from build123d import *

# Parameters (mm, degrees)
BOSS_EXTRUDE1_DEPTH = 23
CUT_EXTRUDE1_REACH  = 53.631
SKETCH4_R           = 1.95
CUT_EXTRUDE3_REACH  = 59.631
CUT_EXTRUDE3_START  = -6
CUT_EXTRUDE4_REACH  = 65.269
SKETCH7_R           = 2.75
CUT_EXTRUDE5_REACH  = 85.269
CUT_EXTRUDE5_START  = -20
SKETCH8_R           = 5
FILLET1_R           = 4


with BuildPart() as part:
    # Sketch3 → Boss-Extrude1 (new, symmetric)
    with BuildSketch(Plane(origin=(0, 0, 0), x_dir=(0, 0, -1), z_dir=(1, 0, 0))):
        Polygon((31.368752944, 7.9863551), (20.770501764, 0), (30, 0), (30, -6), (-30, -6), (-30, 0), (-20.770501764, 0), (16.323377365, 27.952242852), align=None)
    extrude(amount=BOSS_EXTRUDE1_DEPTH, both=True)

    # Sketch4 → Cut-Extrude1 (cut, up to next)
    with BuildSketch(Plane(origin=(0, -6, 0), x_dir=(-1, 0, 0), z_dir=(0, -1, 0)), mode=Mode.PRIVATE) as cut_extrude1_sk1:
        with Locations(Location((15, 15, 0), (0, 0, 90))):
            Circle(SKETCH4_R)
    cut_extrude1_tool1 = extrude(cut_extrude1_sk1.sketch, amount=-CUT_EXTRUDE1_REACH, mode=Mode.PRIVATE) & part.part
    # Sketch4 → Cut-Extrude1 (cut, up to next)
    with BuildSketch(Plane(origin=(0, -6, 0), x_dir=(-1, 0, 0), z_dir=(0, -1, 0)), mode=Mode.PRIVATE) as cut_extrude1_sk2:
        with Locations(Location((15, -15, 0), (0, 0, 90))):
            Circle(SKETCH4_R)
    cut_extrude1_tool2 = extrude(cut_extrude1_sk2.sketch, amount=-CUT_EXTRUDE1_REACH, mode=Mode.PRIVATE) & part.part
    # Sketch4 → Cut-Extrude1 (cut, up to next)
    with BuildSketch(Plane(origin=(0, -6, 0), x_dir=(-1, 0, 0), z_dir=(0, -1, 0)), mode=Mode.PRIVATE) as cut_extrude1_sk3:
        with Locations(Location((-15, -15, 0), (0, 0, 90))):
            Circle(SKETCH4_R)
    cut_extrude1_tool3 = extrude(cut_extrude1_sk3.sketch, amount=-CUT_EXTRUDE1_REACH, mode=Mode.PRIVATE) & part.part
    # Sketch4 → Cut-Extrude1 (cut, up to next)
    with BuildSketch(Plane(origin=(0, -6, 0), x_dir=(-1, 0, 0), z_dir=(0, -1, 0)), mode=Mode.PRIVATE) as cut_extrude1_sk4:
        with Locations(Location((-15, 15, 0), (0, 0, 90))):
            Circle(SKETCH4_R)
    cut_extrude1_tool4 = extrude(cut_extrude1_sk4.sketch, amount=-CUT_EXTRUDE1_REACH, mode=Mode.PRIVATE) & part.part
    add(cut_extrude1_tool1.solids().sort_by_distance((-15, -6, -15))[0], mode=Mode.SUBTRACT)
    add(cut_extrude1_tool2.solids().sort_by_distance((-15, -6, 15))[0], mode=Mode.SUBTRACT)
    add(cut_extrude1_tool3.solids().sort_by_distance((15, -6, 15))[0], mode=Mode.SUBTRACT)
    add(cut_extrude1_tool4.solids().sort_by_distance((15, -6, -15))[0], mode=Mode.SUBTRACT)

    # Sketch6 → Cut-Extrude3 (cut, up to next)
    with BuildSketch(Plane(origin=(0, -6, 0), x_dir=(-1, 0, 0), z_dir=(0, -1, 0)).offset(CUT_EXTRUDE3_START), mode=Mode.PRIVATE) as cut_extrude3_sk1:
        Polygon((-15, -18.983716857), (-18.45, -16.991858429), (-18.45, -13.008141571), (-15, -11.016283143), (-11.55, -13.008141571), (-11.55, -16.991858429), align=None)
    cut_extrude3_tool1 = extrude(cut_extrude3_sk1.sketch, amount=-CUT_EXTRUDE3_REACH, mode=Mode.PRIVATE) & part.part
    # Sketch6 → Cut-Extrude3 (cut, up to next)
    with BuildSketch(Plane(origin=(0, -6, 0), x_dir=(-1, 0, 0), z_dir=(0, -1, 0)).offset(CUT_EXTRUDE3_START), mode=Mode.PRIVATE) as cut_extrude3_sk2:
        Polygon((18.45, -16.991858429), (18.45, -13.008141571), (15, -11.016283143), (11.55, -13.008141571), (11.55, -16.991858429), (15, -18.983716857), align=None)
    cut_extrude3_tool2 = extrude(cut_extrude3_sk2.sketch, amount=-CUT_EXTRUDE3_REACH, mode=Mode.PRIVATE) & part.part
    # Sketch6 → Cut-Extrude3 (cut, up to next)
    with BuildSketch(Plane(origin=(0, -6, 0), x_dir=(-1, 0, 0), z_dir=(0, -1, 0)).offset(CUT_EXTRUDE3_START), mode=Mode.PRIVATE) as cut_extrude3_sk3:
        Polygon((15, 11.016283143), (18.45, 13.008141571), (18.45, 16.991858429), (15, 18.983716857), (11.55, 16.991858429), (11.55, 13.008141571), align=None)
    cut_extrude3_tool3 = extrude(cut_extrude3_sk3.sketch, amount=-CUT_EXTRUDE3_REACH, mode=Mode.PRIVATE) & part.part
    # Sketch6 → Cut-Extrude3 (cut, up to next)
    with BuildSketch(Plane(origin=(0, -6, 0), x_dir=(-1, 0, 0), z_dir=(0, -1, 0)).offset(CUT_EXTRUDE3_START), mode=Mode.PRIVATE) as cut_extrude3_sk4:
        Polygon((-11.733099869, 12.720227307), (-11.392208867, 16.689332159), (-14.659108999, 18.969104852), (-18.266900131, 17.279772693), (-18.607791133, 13.310667841), (-15.340891001, 11.030895148), align=None)
    cut_extrude3_tool4 = extrude(cut_extrude3_sk4.sketch, amount=-CUT_EXTRUDE3_REACH, mode=Mode.PRIVATE) & part.part
    add(cut_extrude3_tool1.solids().sort_by_distance((15, 0, 15))[0], mode=Mode.SUBTRACT)
    add(cut_extrude3_tool2.solids().sort_by_distance((-15, 0, 15))[0], mode=Mode.SUBTRACT)
    add(cut_extrude3_tool3.solids().sort_by_distance((-15, 0, -15))[0], mode=Mode.SUBTRACT)
    add(cut_extrude3_tool4.solids().sort_by_distance((15, 0, -15))[0], mode=Mode.SUBTRACT)

    # Cut-Extrude4: up to this plane
    cut_extrude4_end = Plane(origin=(23, -6, -30), z_dir=(0, 1, 0))
    # Sketch7 → Cut-Extrude4 (cut, up to the surface)
    with BuildSketch(Plane(origin=(0, 17.969298976, -23.846065154), x_dir=(-1, 0, 0), z_dir=(0, 0.6018150231520492, -0.7986355100472922)), mode=Mode.PRIVATE) as cut_extrude4_sk1:
        with Locations(Location((0, 0, 0), (0, 0, 90))):
            Circle(SKETCH7_R)
    cut_extrude4_tool1 = split(extrude(cut_extrude4_sk1.sketch, amount=-CUT_EXTRUDE4_REACH, mode=Mode.PRIVATE), bisect_by=cut_extrude4_end, keep=Keep.BOTH, mode=Mode.PRIVATE)
    add(cut_extrude4_tool1.solids().sort_by_distance((0, 17.969299, -23.846065))[0], mode=Mode.SUBTRACT)

    # Cut-Extrude5: up to this plane
    cut_extrude5_end = Plane(origin=(23, -6, -30), z_dir=(0, 1, 0))
    # Sketch8 → Cut-Extrude5 (cut, up to the surface)
    with BuildSketch(Plane(origin=(0, 17.969298976, -23.846065154), x_dir=(-1, 0, 0), z_dir=(0, 0.6018150231520492, -0.7986355100472922)).offset(CUT_EXTRUDE5_START), mode=Mode.PRIVATE) as cut_extrude5_sk1:
        with Locations(Location((0, 0, 0), (0, 0, 90))):
            Circle(SKETCH8_R)
    cut_extrude5_tool1 = split(extrude(cut_extrude5_sk1.sketch, amount=-CUT_EXTRUDE5_REACH, mode=Mode.PRIVATE), bisect_by=cut_extrude5_end, keep=Keep.BOTH, mode=Mode.PRIVATE)
    add(cut_extrude5_tool1.solids().sort_by_distance((0, 5.932999, -7.873355))[0], mode=Mode.SUBTRACT)

    # Fillet1
    fillet1_edges = [part.edges().sort_by_distance(p)[0] for p in [
        (-23, 13.976121426, 2.2235622),
        (23, -3, 30),
        (23, -3, -30),
        (23, 3.99317755, -26.069627354),
        (23, 13.976121426, 2.2235622),
        (-23, 3.99317755, -26.069627354),
        (-23, -3, -30),
        (-23, -3, 30),
    ]]
    fillet(fillet1_edges, radius=FILLET1_R)


solid = part.part
Can you work these out from the model? Positions are in its coordinate system, mm. A direction names the side the tool comes from. Coordinates: 2 decimals unless noted, no trailing zeros. Write each loop counter-clockwise with the first axis right and the second up, starting at its lowest first coordinate (ties: lowest second). Pieces come first, ordered by that corner, then holes. Notation, with made-up numbers: (58, 3.25) - (103, 3.25) arc R36 cw to (103, 37.25) - close; hole circle Ø8 at (-14, 15). An arc over 180 degrees is marked (long way). Return JSON: item names as keys, results as strings. Group by question number.
Item 1: If we section it at B-B (z = -15): Count the separate pieces of the cut face and the enclosed holes in it, then the cut area to 3 significant figures.
Item 2: Which directions (+Z, -Z, +X, -X, +Y, -Y) give clear straight access to the entire face, cutting with the end or side of a thin tool? Please do faces 1 (the face through (-2.15, 7.65, -6.58)), 2 (the face through (-13.3, 12.5, -12)), 3 (the face through (0.322, 20.327, -22.069)).
Item 3: I'm going to push flat-ended pins straight in: pin 1 Ø3 at (y, z) = (4, 15) entering from +X; pin 2 Ø2 at (x, z) = (-15.5, -16) entering from +Y; pin 3 Ø3 at (x, z) = (-15, -15) entering from +Y; pin 4 Ø4.5 at (y, z) = (1.5, 14) entering from -X. Where does each tip first touch, or does it pass through?
Item 4: If we section it at A-A (x = -7.5): Write out the boundary of the cut face in (y, z).
Item 5: If we section it at C-C (z = 24): Write out the boundary of the cut face in (x, y).
Item 6: Please list where these lines run through material, in increasing order: probe 1 along X at (y, z) = (-1, -15); probe 2 along X at (y, z) = (-2.5, -13.5); probe 3 along Z at (x, y) = (11.5, -0.5).
Item 7: We'd pull the mould along X, two halves only. Please class faces 4 (the face through (21.859, -3.042, -28.797)), 5 (the face through (5, -6, 0)), 6 (the face through (-11.55, 2, 15)): pulls with the +X half, pulls with the -X half, needs draft (parallel to the pull), parting line crosses it, or undercut.
Return value:
{
 "1": {"separate pieces": "3", "enclosed holes": "1", "area": "1,060 mm^2"},
 "2": {"face 1": "none", "face 2": "+Y", "face 3": "-Z, +X, -X, +Y"},
 "3": {"pin 1": "stops at x = 22.33", "pin 2": "stops at y = 0", "pin 3": "passes through", "pin 4": "stops at x = -23"},
 "4": {"outline": "(-6, -30) - (0, -30) - (0, -20.77) - (7.99, -31.37) - (27.95, -16.32) - (0, 20.77) - (0, 30) - (-6, 30) - close"},
 "5": {"outline": "(-23, -6) - (23, -6) - (23, 0) - (-23, 0) - close"},
 "6": {"probe 1": "x = -23 to -16.95, -13.05 to 13.05, 16.95 to 23", "probe 2": "x = -23 to -16.25, -13.75 to 13.75, 16.25 to 23", "probe 3": "z = -30 to 30"},
 "7": {"face 4": "pulls with the +X half", "face 5": "needs draft", "face 6": "undercut"}
}
